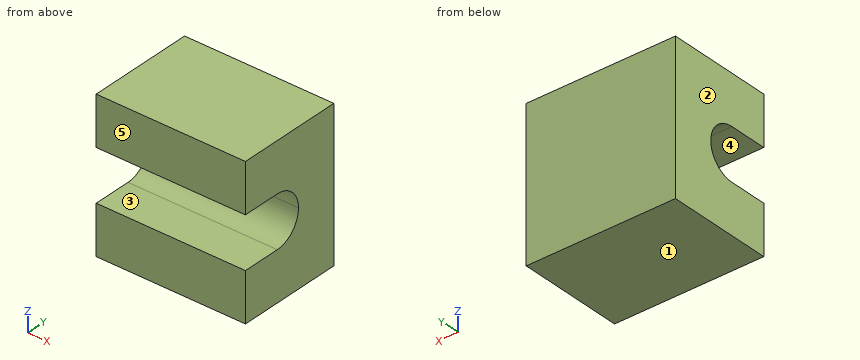
from build123d import *

# Parameters (mm, degrees)
BOSS_EXTRUDE1_DEPTH = 35


with BuildPart() as part:
    # Sketch1 → Boss-Extrude1 (new body)
    with BuildSketch(Plane(origin=(0, 0, 0), x_dir=(0, 0, -1), z_dir=(1, 0, 0))):
        with BuildLine():
            Line((-8.82183908, 6.781609195), (-8.82183908, 16.781609195))
            Line((-8.82183908, 16.781609195), (-26.32183908, 16.781609195))
            Line((-26.32183908, 16.781609195), (-26.32183908, -8.218390805))
            Line((-26.32183908, -8.218390805), (-14.82183908, -8.218390805))
            Line((-14.82183908, -8.218390805), (-14.82183908, 0.781609195))
            ThreePointArc((-14.82183908, 0.781609195), (-13.064479768, 5.024249883), (-8.82183908, 6.781609195))
        make_face()
        with BuildLine():
            Line((8.67816092, 16.781609195), (-8.82183908, 16.781609195))
            Line((-8.82183908, 16.781609195), (-8.82183908, 6.781609195))
            ThreePointArc((-8.82183908, 6.781609195), (-4.579198393, 5.024249883), (-2.82183908, 0.781609195))
            Line((-2.82183908, 0.781609195), (-2.82183908, -8.218390805))
            Line((-2.82183908, -8.218390805), (8.67816092, -8.218390805))
            Line((8.67816092, -8.218390805), (8.67816092, 16.781609195))
        make_face()
    extrude(amount=BOSS_EXTRUDE1_DEPTH)


solid = part.part
Design review of the part built by this model. Coordinates are the model's own, in mm. Face numbers are marked on the shaded views. A direction names the side the tool comes from. Give positions to 0.01 mm unless a question says otherwise; leave off trailing zeros. Write each loop counter-clockwise with the first axis right and the second up, starting at its lowest first coordinate (ties: lowest second). Pieces come first, ordered by that corner, then holes. Notation, with made-up numbers: M 3,37.5 L 23,37.5 A27 cw 23,75.5 Z; hole C -14,54.25 d7. An arc over 180 degrees is marked long. Answer as a JSON object with one key per item and string values. Group by question number.
1) We need section B-B (x = 24). Give the boundary of the cut face in (y, z).
2) We need section A-A (y = -6.25). Give the boundary of the cut face in (x, z), and give its area (3 significant figures).
3) Tool access review of the marked faces 4 and 5: name each direction out of +Z, -Z, +X, -X, +Y, -Y from which nothing blocks a thin tool from reaching the whole face with its end or side.
4) Mouldability with a two-part tool opening along Z and no side actions: class the marked faces 1, 2 and 3 as released by +Z, released by -Z, zero draft, split by the parting line, or undercut.
5) We need section C-C (z = 13.5). Give the boundary of the cut face in (x, y).
6) For line 1 along Z through (x, y) = (4.5, -4.25); line 2 along Z through (x, y) = (16, 5.5); line 3 along Y through (x, z) = (13.5, 6), list the stretches that pass through material, from the lowest coordinate up.
Answer key:
{
 "1": {"outline": "M -8.22,-8.68 L 16.78,-8.68 L 16.78,26.32 L -8.22,26.32 L -8.22,14.82 L 0.78,14.82 A6 cw 0.78,2.82 L -8.22,2.82 Z"},
 "2": {"outline": "M 0,-8.68 L 35,-8.68 L 35,2.82 L 0,2.82 Z; M 0,14.82 L 35,14.82 L 35,26.32 L 0,26.32 Z", "area": "805 mm²"},
 "3": {"face 4": "+X, -X, -Y", "face 5": "+Z, -Z, +X, -X, -Y"},
 "4": {"face 1": "released by -Z", "face 2": "zero draft", "face 3": "undercut"},
 "5": {"outline": "M 0,4.54 L 35,4.54 L 35,16.78 L 0,16.78 Z"},
 "6": {"line 1": "z = -8.68 to 2.82, 14.82 to 26.32", "line 2": "z = -8.68 to 5.12, 12.53 to 26.32", "line 3": "y = 6.08 to 16.78"}
}
